```python
from build123d import *

# Parameters (mm, degrees)
BOX001_W               = 10
BOX001_H               = 2.5
BOX001_DEPTH           = 10
BOX001_PLACEMENT_ANGLE = 135
BOX_W                  = 10
BOX_H                  = 2.5
BOX_DEPTH              = 10
BOX_ROLL_ANGLE         = 45
TORUS_R                = 5
TORUS_PITCH_ANGLE      = 90


with BuildPart() as obj1:
    # Box001 → Box001 (new body)
    with BuildSketch(Plane.XY):
        with Locations((5, 1.25)):
            Rectangle(BOX001_W, BOX001_H)
    extrude(amount=BOX001_DEPTH)


with BuildPart() as obj1_1:
    # Box001 placement: moved
    add(obj1.part.moved(Location((25, -14.580583, -17.632621))).rotate(Axis((25, -14.580583, -17.632621), (1, 0, 0)), BOX001_PLACEMENT_ANGLE))


with BuildPart() as obj2:
    # Box → Box (new body)
    with BuildSketch(Plane.XY):
        with Locations((5, 1.25)):
            Rectangle(BOX_W, BOX_H)
    extrude(amount=BOX_DEPTH)


with BuildPart() as obj2_1:
    # Box roll: moved
    add(obj2.part.rotate(Axis((0, 0, 0), (1, 0, 0)), BOX_ROLL_ANGLE))


with BuildPart() as obj2_2:
    # Box placement: moved
    add(obj2_1.part.moved(Location((25, -16.34835, -24.703689))))


with BuildPart() as obj3:
    # Torus → Torus (revolve)
    with BuildSketch(Plane.XZ):
        with Locations((20, 0)):
            Circle(TORUS_R)
    revolve(axis=Axis((0, 0, 0), (0, 0, 1)))


with BuildPart() as obj3_1:
    # Torus pitch: moved
    add(obj3.part.rotate(Axis((0, 0, 0), (0, 1, 0)), TORUS_PITCH_ANGLE))


with BuildPart() as obj3_2:
    # Torus placement: moved
    add(obj3_1.part.moved(Location((0, 0, 50))))


with BuildPart() as obj4:
    # Sphere001 → Sphere001 (revolve)
    with BuildSketch(Plane(origin=(40, -20, -20), x_dir=(1, 0, 0), z_dir=(0, -1, 0))):
        with BuildLine():
            ThreePointArc((0, -10), (10, 0), (0, 10))
            Line((0, 10), (0, -10))
        make_face()
    revolve(axis=Axis((40, -20, -20), (0, 0, 1)))


with BuildPart() as cut002:
    # Sphere → Sphere (revolve)
    with BuildSketch(Plane.XZ):
        with BuildLine():
            ThreePointArc((0, -50), (50, 0), (0, 50))
            Line((0, 50), (0, -50))
        make_face()
    revolve(axis=Axis((0, 0, 0), (0, 0, 1)))

    # Cut: cut obj4
    add(obj4.part, mode=Mode.SUBTRACT)

    # Fusion: union obj3
    add(obj3_2.part)

    # Cut001: cut obj2
    add(obj2_2.part, mode=Mode.SUBTRACT)

    # Cut002: cut obj1
    add(obj1_1.part, mode=Mode.SUBTRACT)


solid = cut002.part
```
Verification items for the finished model (mm, model axes). Coordinates: 2 decimals unless noted, no trailing zeros. Loops run counter-clockwise (first coordinate to the right, second up) from the corner with the lowest first, then second, coordinate; pieces in that order, holes last. Notation, with made-up numbers: (59.25, 3) -> (116.25, 3) arc R22 cw to (116.25, 14) -> close; hole circle Ø8 at (-5.5, 56). An arc over 180 degrees is marked (long way). Answer in a Markdown table with one row per item. Add a question column.
1. Section check D-D, the plane y = -27. Enter the section's corners in (x, z).
2. Section check A-A, the plane z = -1. Enter the section's corners in (x, y).
3. Section check C-C, the plane x = 37. Enter the section's corners in (y, z).
4. Section check B-B, the plane y = 33. Enter the section's corners in (x, z), then the cut area to 3 significant figures.
5. Depth check by flat-ended pin: P1, Ø12, axis at x = -8, y = 23.5, coming from the -Z side; P2, Ø3, axis at y = -26.5, z = -14, coming from the -X side; P3, Ø10, axis at y = 39.5, z = -13, coming from the -X side; P4, Ø8, axis at y = -39, z = 42.5, coming from the -X side. Enter the tip coordinate at first touch or a pass-through.
6. Material ranges on probe 1 along Z at (x, y) = (-42, -17); probe 2 along X at (y, z) = (-17, -3.5); probe 3 along Z at (x, y) = (13, 26), recorded low to high. Write a range as [from, to].
Derived:
| question | item | result |
|---|---|---|
| 1 | outline | (34.33, -24.34) arc R7.14 cw to (40.07, -12.86) arc R42.08 ccw (long way) to start |
| 2 | outline | circle Ø99.98 at (0, 0) |
| 3 | outline | (-29.04, -16.96) arc R9.54 cw (long way) to (-16.96, -29.04) arc R33.63 ccw (long way) to start |
| 4 | outline | circle Ø75.13 at (0, 0) |
| 4 | area | 4,430 mm² |
| 5 | P1 | stops at z = -46.32 |
| 5 | P2 | stops at x = -41.1 |
| 5 | P3 | stops at x = -34.08 |
| 5 | P4 | passes through |
| 6 | probe 1 | z = [-21.14, 21.14] |
| 6 | probe 2 | x = [-46.89, 46.89] |
| 6 | probe 3 | z = [-40.68, 40.68] |
